Could you check a few things on this model? Use its own coordinates, in mm. Coordinates: 2 decimals unless noted, no trailing zeros. Order: outer loops, then holes, each group sorted by start corner. A loop starts at its lowest first (then second) coordinate and runs counter-clockwise, first axis right, second up. Notation, with made-up numbers: (-6, 84.25) - (48, 84.25) arc R23 cw to (48, 107.25) - close; hole circle Ø1 at (33.25, 44.25). An arc over 180 degrees is marked (long way). One line per item, written item: value.
from build123d import *

# Parameters (mm, degrees)
BOSS_EXTRUDE1_DEPTH = 3.175
SKETCH2_R           = 3.175
CUT_EXTRUDE1_DEPTH  = 48.961405128


with BuildPart() as part:
    # Sketch1 → Boss-Extrude1 (new body)
    with BuildSketch(Plane.XY):
        with BuildLine():
            Line((-28.328951223, 3.070773738), (-28.328951223, -35.029226262))
            ThreePointArc((-28.328951223, -35.029226262), (-27.399015253, -37.274290292), (-25.153951223, -38.204226262))
            Line((-25.153951223, -38.204226262), (25.646048777, -38.204226262))
            ThreePointArc((25.646048777, -38.204226262), (27.891112807, -37.274290292), (28.821048777, -35.029226262))
            Line((28.821048777, -35.029226262), (28.821048777, 3.070773738))
            ThreePointArc((28.821048777, 3.070773738), (27.891112807, 5.315837768), (25.646048777, 6.245773738))
            Line((25.646048777, 6.245773738), (-25.153951223, 6.245773738))
            ThreePointArc((-25.153951223, 6.245773738), (-27.399015253, 5.315837768), (-28.328951223, 3.070773738))
        make_face()
    extrude(amount=-BOSS_EXTRUDE1_DEPTH)

    # Sketch2 → Cut-Extrude1 (cut, through all)
    with BuildSketch(Plane.XY):
        with Locations((-17.152951223, -5.184226262)):
            Circle(SKETCH2_R)
        with Locations(Location((17.645048777, -5.184226262, 0), (0, 0, 180))):
            Circle(SKETCH2_R)
    extrude(amount=-CUT_EXTRUDE1_DEPTH, mode=Mode.SUBTRACT)


solid = part.part
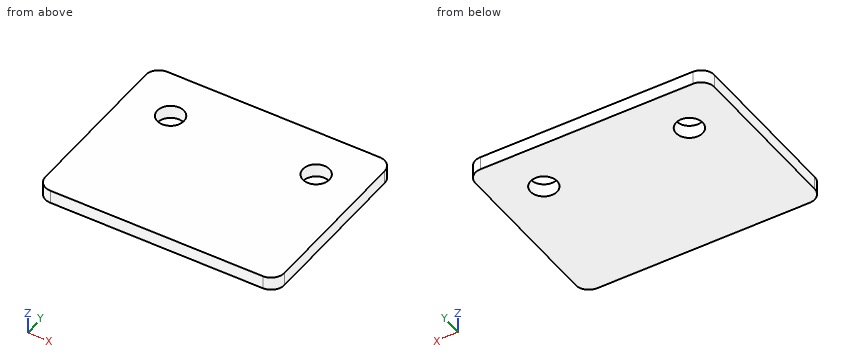
Item 1: I'm going to push a flat-ended pin straight in: pin 1 Ø4 at (x, y) = (22, -17) entering from +Z. Where does the tip first touch, or does it pass through?
Conclusion:
pin 1: z = 0
Item 2: If I drill on probe 1 along Y at (x, z) = (17.5, -0.9); probe 2 along X at (y, z) = (-5.5, -2.5); probe 3 along X at (y, z) = (-7, -2.55), over which ranges is the centre line in solid material (lowest first)?
Conclusion:
probe 1: -38.2 to -8.36, -2.01 to 6.25
probe 2: -28.33 to -20.31, -13.99 to 14.49, 20.8 to 28.82
probe 3: -28.33 to -19.76, -14.55 to 15.04, 20.25 to 28.82
Item 3: I want a section at B-B on z = -2.5. Please give me the cut outline in (x, y) (3 decimals), then the cut area to 3 significant figures.
Conclusion:
outline: (-28.329, -35.029) arc R3.175 ccw to (-25.154, -38.204) - (25.646, -38.204) arc R3.175 ccw to (28.821, -35.029) - (28.821, 3.071) arc R3.175 ccw to (25.646, 6.246) - (-25.154, 6.246) arc R3.175 ccw to (-28.329, 3.071) - close; hole circle Ø6.35 at (-17.153, -5.184); hole circle Ø6.35 at (17.645, -5.184)
area: 2,470 mm²
Item 4: I want a section at A-A on x = 17.5. Please give me the cut outline in (y, z) (3 decimals), then the cut area to 3 significant figures.
Conclusion:
outline: (-38.204, -3.175) - (-8.356, -3.175) - (-8.356, 0) - (-38.204, 0) - close; (-2.013, -3.175) - (6.246, -3.175) - (6.246, 0) - (-2.013, 0) - close
area: 121 mm²
